Input: dimensioned drawing with shaded views. Units: mm. Origin: part minimum x, y, z. A direction names the side the tool comes from. Round coordinates to 2 decimals unless told otherwise and drop trailing zeros. Order: outer loops, then holes, each group sorted by start corner. A loop starts at its lowest first (then second) coordinate and runs counter-clockwise, first axis right, second up. Notation, with made-up numbers: M 85,58.25 L 123,58.25 A15 cw 123,65.25 Z; hole C 26,-8 d7. An arc over 180 degrees is marked long. One line per question, with ' | ' between items.
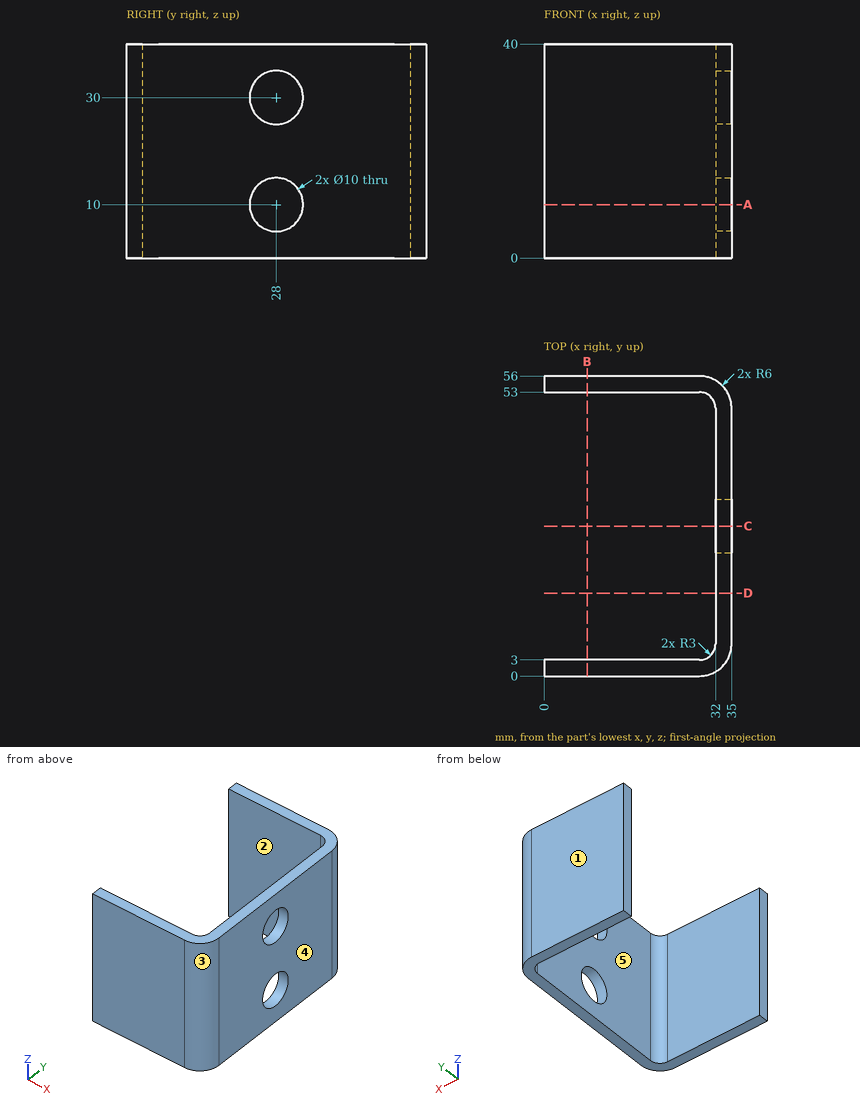
Item 1: Section query A-A, the plane z = 10. Return loops of the section in (x, y).
Report:
outline: M 0,0 L 29,0 A6 ccw 35,6 L 35,23 L 32,23 L 32,6 A3 cw 29,3 L 0,3 Z; M 0,53 L 29,53 A3 cw 32,50 L 32,33 L 35,33 L 35,50 A6 ccw 29,56 L 0,56 Z
Item 2: Section query D-D, the plane y = 15.5. Return loops of the section in (x, z), plus the area to 3 significant figures.
Report:
outline: M 32,0 L 35,0 L 35,40 L 32,40 Z | area: 120 mm²
Item 3: Section query B-B, the plane x = 8. Return loops of the section in (y, z), plus the area to 3 significant figures.
Report:
outline: M 0,0 L 3,0 L 3,40 L 0,40 Z; M 53,0 L 56,0 L 56,40 L 53,40 Z | area: 240 mm²
Item 4: Section query C-C, the plane y = 28. Return loops of the section in (x, z).
Report:
outline: M 32,0 L 35,0 L 35,5 L 32,5 Z; M 32,15 L 35,15 L 35,25 L 32,25 Z; M 32,35 L 35,35 L 35,40 L 32,40 Z
Item 5: Line query: line 1 along Y through (x, z) = (27.5, 5); line 2 along Z through (x, y) = (33.5, 28.5); line 3 along X through (y, z) = (43, 17). Output: solid intervals per line, ascending. Write a range as from..to.
Report:
line 1: 0..3, 53..56 | line 2: 0..5.03, 14.97..25.03, 34.97..40 | line 3: 32..35
Item 6: Access query for the marked faces 1 and 2. Directions: +Z, -Z, +X, -X, +Y, -Y. A direction counts if a zero-diameter tool reaches every point of the face in a straight line with its end or side. Return the directions, or none.
Report:
face 1: +Z, -Z, +X, -X, +Y | face 2: +Z, -Z, -X
Item 7: Mould query, pull axis Y, two halves, no side actions, for the marked faces 3, 4 and 5. Classes: +Y half, -Y half, draft (parallel to the pull), parting line (faces both ways), or undercut.
Report:
face 3: -Y half | face 4: draft | face 5: undercut
Item 8: First-contact query: pin 1 (20 mm diameter, centred on y = 32.5, z = 17, fed in from -X). Flat tip, straight axial feed; report the tip coordinate or a pass-through.
Report:
pin 1: x = 32
